```python
from build123d import *

# Parameters (mm, degrees)
F0_W     = 12.3444
F0_H     = 22.7584
F0_R     = 1.651
F1_DEPTH = 3.175


# Not quite as in the source:
# - a length typed as a fraction of an inch, garbled in the dataset ("3 / 203.2 mm" for 3/8 in), is restored


with BuildPart() as f1:
    # F0 (on Top) → F1 (new body)
    with BuildSketch(Plane.XY):
        Polygon((0, 86.4107935882), (0, 0), (19.2153378795, 0), (88.9, 0), (88.9, 15.8380966835), (88.9, 86.4107935882), (76.3653378795, 86.4107935882), (76.3653378795, 15.8380966835), (19.2153378795, 15.8380966835), (19.2153378795, 86.4107935882), align=None)
        with Locations((9.3165273066, 24.6552514774)):
            Rectangle(F0_W, F0_H, mode=Mode.SUBTRACT)
        with Locations((9.3165273066, 67.1494514774)):
            Circle(F0_R, mode=Mode.SUBTRACT)
    extrude(amount=F1_DEPTH)


solid = f1.part
```
Geometry: final body of the model. Coordinates: model frame, mm. A direction names the side the tool comes from. Give positions to 0.01 mm unless a question says otherwise; leave off trailing zeros. Order: outer loops, then holes, each group sorted by start corner. A loop starts at its lowest first (then second) coordinate and runs counter-clockwise, first axis right, second up. Notation, with made-up numbers: (-1, 75) -> (15, 75) arc R23 cw to (15, 104) -> close; hole circle Ø9 at (82, 29.5). An arc over 180 degrees is marked (long way). Write each question's results on one line, items separated by ' | '. Start each with the question number.
1) Draft query along X for faces 4 (the flat face through (9, 36.034, 2)), 5 (the flat face through (0, 44, 2)), 6 (the flat face through (83, 86.411, 2)), 7 (the flat face through (88.9, 43, 2)). Return one class per face: pulls with the +X half, pulls with the -X half, needs draft (parallel to the pull), parting line crosses it, or undercut.
2) Section B-B (z = 1.1). Return loops of the section in (x, y).
3) Set-up query: faces 1 (the flat face through (3.144, 24, 2)), 2 (the flat face through (10, 86.411, 2)), 3 (the flat face through (48, 15.838, 2)). Return all of +Z, -Z, +X, -X, +Y, -Y with unobstructed straight access to the full face (end or side cutting, diameter ignored); none if empty.
4) Line query: line 1 (X direction, y = 30.5, z = 1.8); line 2 (X direction, y = 76, z = 2.25); line 3 (Y direction, x = 9, z = 2). Output: solid intervals per line, ascending. Write a range as from..to.
5) Section A-A (y = 56). Return loops of the section in (x, z) (3 decimals).
6) Section C-C (x = 71). Return loops of the section in (y, z) (3 decimals), then the cut area to 3 significant figures.
7) First-contact query: pin 1 (5 mm diameter, centred on x = 24, y = 38.5, fed in from -Z); pin 2 (5.5 mm diameter, centred on x = 9.32, y = 67.15, fed in from +Z) (3 decimals). Flat tips, straight axial feed; report the tip coordinate or a pass-through.
Calculated:
1) face 4: undercut | face 5: pulls with the -X half | face 6: needs draft | face 7: pulls with the +X half
2) outline: (0, 0) -> (88.9, 0) -> (88.9, 86.41) -> (76.37, 86.41) -> (76.37, 15.84) -> (19.22, 15.84) -> (19.22, 86.41) -> (0, 86.41) -> close; hole (3.14, 13.28) -> (15.49, 13.28) -> (15.49, 36.03) -> (3.14, 36.03) -> close; hole circle Ø3.3 at (9.32, 67.15)
3) face 1: +Z, -Z | face 2: +Z, -Z, +X, -X, +Y | face 3: +Z, -Z, +Y
4) line 1: 0..3.14, 15.49..19.22, 76.37..88.9 | line 2: 0..19.22, 76.37..88.9 | line 3: 0..13.28, 36.03..65.53, 68.77..86.41
5) outline: (0, 0) -> (19.215, 0) -> (19.215, 3.175) -> (0, 3.175) -> close; (76.365, 0) -> (88.9, 0) -> (88.9, 3.175) -> (76.365, 3.175) -> close
6) outline: (0, 0) -> (15.838, 0) -> (15.838, 3.175) -> (0, 3.175) -> close | area: 50.3 mm2
7) pin 1: through | pin 2: z = 3.175
